Source: CAD feature listing. Evaluate the final solid. Frame: model axes, mm. Round coordinates to 2 decimals unless told otherwise and drop trailing zeros. Order: outer loops, then holes, each group sorted by start corner. A loop starts at its lowest first (then second) coordinate and runs counter-clockwise, first axis right, second up. Notation, with made-up numbers: (87.25, 22) - (124.25, 22) arc R18 ccw to (124.25, 53) - close; hole circle Ø8 at (88, 78). An arc over 180 degrees is marked (long way). Use one line per item in the form item = value. Start each with the question number.
Q1. Cut plane A-A, the plane z = 3.15. Return the cut outline in (x, y).
Q2. Pin query (flat end, axial travel): pin 1 Ø2 at (x, z) = (-92, 2) entering from -Y; pin 2 Ø2 at (y, z) = (-49, 1) entering from +X; pin 3 Ø1.2 at (x, z) = (-51.5, 1.5) entering from -Y. Return the tip coordinate at first contact, or that it passes through.
Q3. Cut plane D-D, the plane x = -40. Return the cut outline in (y, z).
Q4. Cut plane B-B, the plane x = 15. Return the cut outline in (y, z), and give its area (3 significant figures).
Q5. Cut plane C-C, the plane y = -57. Return the cut outline in (x, z).
Q6. Ray query, line 1 (X direction, y = -61, z = 1.75); line 2 (X direction, y = -40, z = 1.65); line 3 (Y direction, x = -43.5, z = 3.2). Return the intervals inside material, ascending. Write a range as [from, to].
from build123d import *

# Parameters (mm, degrees)
F1_DEPTH = 4.064
F2_W     = 25.4
F2_H     = 3.0734
F3_DEPTH = 25.4


with BuildPart() as f1:
    # F0 (on Top) → F1 (new body)
    with BuildSketch(Plane.XY):
        with BuildLine():
            Line((-93.431173, -62.185294), (-93.431173, -74.885294))
            ThreePointArc((-93.431173, -74.885294), (-17.231173, -66.45046), (58.968827, -74.885294))
            Line((58.968827, -74.885294), (58.968827, -62.185294))
            Line((58.968827, -62.185294), (54.904827, -62.185294))
            Line((54.904827, -62.185294), (54.904827, -38.944294))
            Line((54.904827, -38.944294), (58.968827, -38.944294))
            Line((58.968827, -38.944294), (58.968827, -36.785294))
            Line((58.968827, -36.785294), (58.968827, -26.244294))
            Line((58.968827, -26.244294), (54.904827, -26.244294))
            Line((54.904827, -26.244294), (-93.431173, -26.244294))
            Line((-93.431173, -26.244294), (-93.431173, -38.944294))
            Line((-93.431173, -38.944294), (-89.367173, -38.944294))
            Line((-89.367173, -38.944294), (-89.367173, -62.185294))
            Line((-89.367173, -62.185294), (-93.431173, -62.185294))
        make_face()
    extrude(amount=F1_DEPTH)

    # F2 (on face) → F3 (cut)
    with BuildSketch(Plane.XY.offset(4.064)):
        with Locations((20.868827, -62.386453)):
            Rectangle(F2_W, F2_H)
        with Locations((-55.331173, -62.386453)):
            Rectangle(F2_W, F2_H)
    extrude(amount=-F3_DEPTH, mode=Mode.SUBTRACT)


solid = f1.part
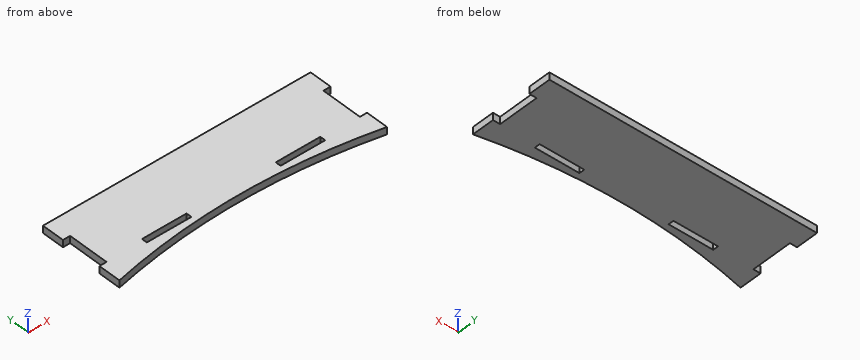
Completed:
q1.outline = (-93.43, -74.89) arc R348.41 cw to (58.97, -74.89) - (58.97, -62.19) - (54.9, -62.19) - (54.9, -38.94) - (58.97, -38.94) - (58.97, -26.24) - (-93.43, -26.24) - (-93.43, -38.94) - (-89.37, -38.94) - (-89.37, -62.19) - (-93.43, -62.19) - close; hole (-68.03, -63.92) - (-42.63, -63.92) - (-42.63, -60.85) - (-68.03, -60.85) - close; hole (8.17, -63.92) - (33.57, -63.92) - (33.57, -60.85) - (8.17, -60.85) - close
q2.pin_1 = -74.79
q2.pin_2 = 54.9
q2.pin_3 = -68.2
q3.outline = (-67.2, 0) - (-26.24, 0) - (-26.24, 4.06) - (-67.2, 4.06) - close
q4.outline = (-67.94, 0) - (-63.92, 0) - (-63.92, 4.06) - (-67.94, 4.06) - close; (-60.85, 0) - (-26.24, 0) - (-26.24, 4.06) - (-60.85, 4.06) - close
q4.area = 157 mm2
q5.outline = (-89.37, 0) - (54.9, 0) - (54.9, 4.06) - (-89.37, 4.06) - close
q6.line_1 = [-89.37, -68.03], [-42.63, 8.17], [33.57, 54.9]
q6.line_2 = [-89.37, 54.9]
q6.line_3 = [-67.44, -63.92], [-60.85, -26.24]
